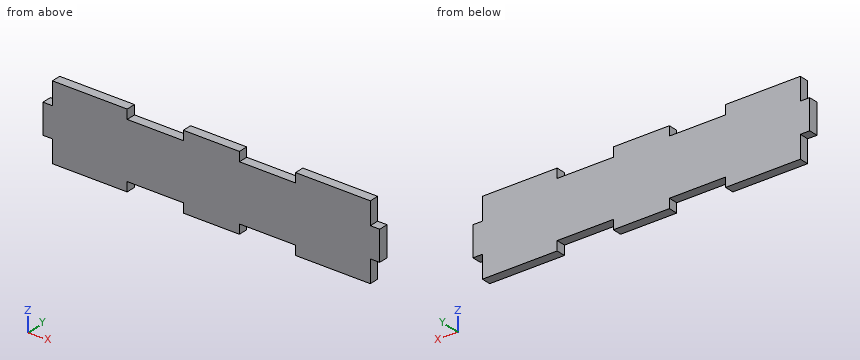
Autodesk Inventor part; units mm, degrees
ref_plane "YZ Plane" through (0, 0, 0) normal (1, 0, 0) x (0, 1, 0)
ref_plane "XZ Plane" through (0, 0, 0) normal (0, 1, 0) x (-1, 0, 0)
ref_plane "XY Plane" through (0, 0, 0) normal (0, 0, 1) x (1, 0, 0)
sketch "Sketch1" plane through (0, 0, 0) normal (0, 1, 0) x (-1, 0, 0)
  line L0 (10.3774, 19.343) -> (-159.6226, 19.343)
  line L1 (-159.6226, 19.343) -> (-159.6226, -20.657)
  line L2 (-159.6226, -20.657) -> (10.3774, -20.657)
  line L3 (10.3774, -20.657) -> (10.3774, 19.343)
  line L4 (10.3774, 7.343) -> (15.3774, 7.343)
  line L5 (15.3774, 7.343) -> (15.3774, -8.657)
  line L6 (15.3774, -8.657) -> (10.3774, -8.657)
  line L7 (10.3774, -8.657) -> (10.3774, 7.343)
  line L8 (-159.6226, 7.343) -> (-164.6226, 7.343)
  line L9 (-164.6226, 7.343) -> (-164.6226, -8.657)
  line L10 (-164.6226, -8.657) -> (-159.6226, -8.657)
  line L11 (-159.6226, -8.657) -> (-159.6226, 7.343)
  line L12 (-119.6226, -20.657) -> (-89.6226, -20.657)
  line L13 (-89.6226, -20.657) -> (-89.6226, -15.657)
  line L14 (-89.6226, -15.657) -> (-119.6226, -15.657)
  line L15 (-119.6226, -15.657) -> (-119.6226, -20.657)
  line L16 (-59.6226, -20.657) -> (-29.6226, -20.657)
  line L17 (-29.6226, -20.657) -> (-29.6226, -15.657)
  line L18 (-29.6226, -15.657) -> (-59.6226, -15.657)
  line L19 (-59.6226, -15.657) -> (-59.6226, -20.657)
  line L20 (-159.6226, -0.657) -> (10.3774, -0.657) construction
  line L21 (-74.6226, 19.343) -> (-74.6226, -20.657) construction
  line L22 (-89.6226, 19.343) -> (-89.6226, 14.343)
  line L23 (-89.6226, 14.343) -> (-119.6226, 14.343)
  line L24 (-119.6226, 14.343) -> (-119.6226, 19.343)
  line L25 (-29.6226, 19.343) -> (-29.6226, 14.343)
  line L26 (-29.6226, 14.343) -> (-59.6226, 14.343)
  line L27 (-59.6226, 14.343) -> (-59.6226, 19.343)
  line L28 (-74.6226, -20.657) -> (-74.6226, 19.343) construction
  point P0 (0, 0)
  point P1 (10.3774, -8.657)
  point P2 (-159.6226, -8.657)
  point P3 (-89.6226, -20.657)
  point P4 (-29.6226, -20.657)
  point P5 (-29.6226, 19.343)
  point P6 (-59.6226, 19.343)
  point P7 (-89.6226, 19.343)
  point P8 (-119.6226, 19.343)
  dimension "d0" = 170
  dimension "d1" = 40
  dimension "d2" = 5
  dimension "d3" = 16
  dimension "d4" = 12
  dimension "d5" = 5
  dimension "d6" = 16
  dimension "d7" = 12
  dimension "d17" = 30
  dimension "d18" = 5
  dimension "d19" = 30
  dimension "d20" = 30
  dimension "d21" = 15
extrude "Extrusion1" add sketch "Sketch1" along normal blind 5 contours L3 L2 L17 L18 L19 L13 L14 L15 L1 L0 L24 L23 L22 L27 L26 L25 | L4 L5 L6 L3 | L1 L10 L9 L8
equation "\"d3\" = d6"
equation "\"d7\" = d4"
properties part number "Superior 1"
Check sheet for the modelled part. Datum: model origin and axes. Units: mm. Round coordinates to 2 decimals unless told otherwise and drop trailing zeros. Loops run counter-clockwise (first coordinate to the right, second up) from the corner with the lowest first, then second, coordinate; pieces in that order, holes last. Notation, with made-up numbers: (27.5, 34) - (79.5, 34) arc R31 ccw to (79.5, 71) - close; hole circle Ø9 at (-4, 87.25). An arc over 180 degrees is marked (long way). Answer as a JSON object with one key per item and string values. Group by question number.
Q1. Sectioned sample at A-A, the plane y = 1.4. Enter the section's corners in (x, z).
Q2. Scan lines: line 1 along X through (y, z) = (4.1, -18); line 2 along X through (y, z) = (1.1, -12.5); line 3 along Z through (x, y) = (94, 0.8). Record each from-to range of solid material in increasing order. Write a range as [from, to].
Q3. Gauge pin test, flat ends, axial feed: P1, Ø2.5, axis at y = 1.5, z = -19, coming from the -X side; P2, Ø1.5, axis at x = 101, y = 1.5, coming from the -Z side; P3, Ø2.5, axis at y = 3, z = 11, coming from the +X side. Record the tip position at first contact, or that the pin passes through.
Q4. Sectioned sample at B-B, the plane x = 45.5. Enter the section's corners in (y, z).
Q5. Sectioned sample at C-C, the plane z = 10. Enter the section's corners in (x, y).
Solution:
{
 "1": {"outline": "(-15.38, -8.66) - (-10.38, -8.66) - (-10.38, -20.66) - (29.62, -20.66) - (29.62, -15.66) - (59.62, -15.66) - (59.62, -20.66) - (89.62, -20.66) - (89.62, -15.66) - (119.62, -15.66) - (119.62, -20.66) - (159.62, -20.66) - (159.62, -8.66) - (164.62, -8.66) - (164.62, 7.34) - (159.62, 7.34) - (159.62, 19.34) - (119.62, 19.34) - (119.62, 14.34) - (89.62, 14.34) - (89.62, 19.34) - (59.62, 19.34) - (59.62, 14.34) - (29.62, 14.34) - (29.62, 19.34) - (-10.38, 19.34) - (-10.38, 7.34) - (-15.38, 7.34) - close"},
 "2": {"line 1": "x = [-10.38, 29.62], [59.62, 89.62], [119.62, 159.62]", "line 2": "x = [-10.38, 159.62]", "line 3": "z = [-15.66, 14.34]"},
 "3": {"P1": "stops at x = -10.38", "P2": "stops at z = -15.66", "P3": "stops at x = 159.62"},
 "4": {"outline": "(0, -15.66) - (5, -15.66) - (5, 14.34) - (0, 14.34) - close"},
 "5": {"outline": "(-10.38, 0) - (159.62, 0) - (159.62, 5) - (-10.38, 5) - close"}
}
